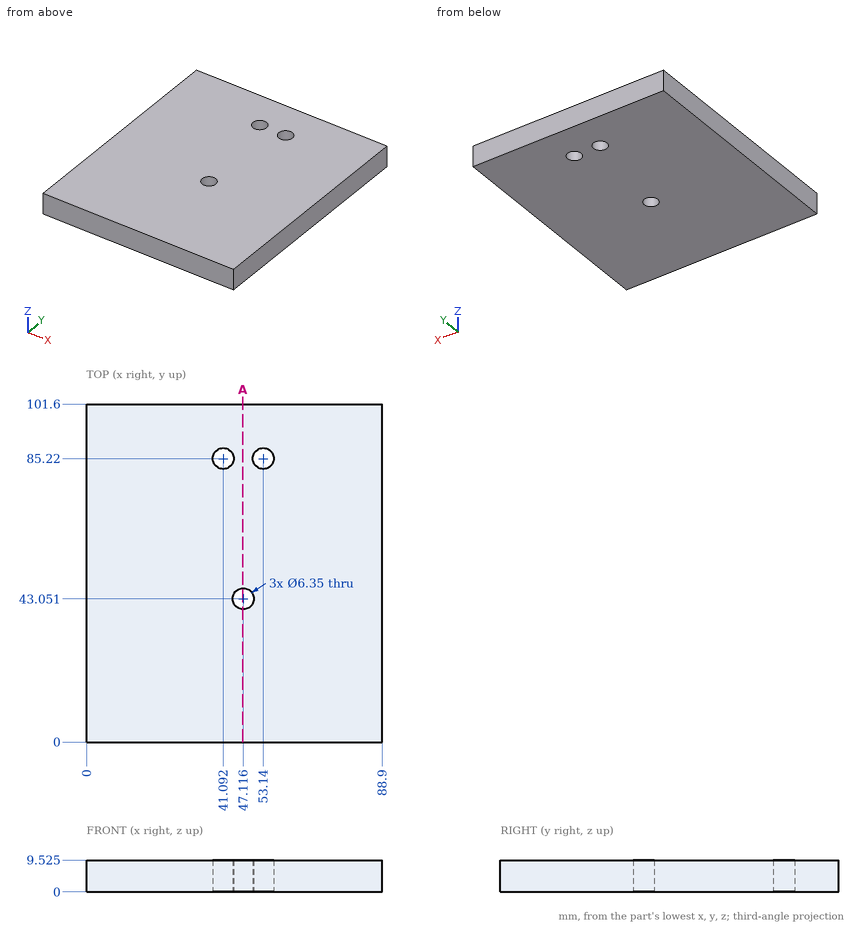
Check sheet for the drawn part. Datum: minimum x, y, z corner. Units: mm. Round coordinates to 2 decimals unless told otherwise and drop trailing zeros. Write each loop counter-clockwise with the first axis right and the second up, starting at its lowest first coordinate (ties: lowest second). Pieces come first, ordered by that corner, then holes. Notation, with made-up numbers: (12.5, 41) -> (58.5, 41) arc R30 ccw to (58.5, 66) -> close; hole circle Ø5 at (-20.75, 74.25). An arc over 180 degrees is marked (long way). Write each question's results on one line, items separated by ' | '. Start each with the question number.
1. Material ranges on probe 1 along X at (y, z) = (85, 4.25) (1 decimal); probe 2 along X at (y, z) = (88, 8.75) (1 decimal); probe 3 along X at (y, z) = (43, 6.5), recorded low to high. Write a range as from..to.
2. Cross-section at A-A (x = 47). Enter the section's corners in (y, z) (1 decimal).
3. Depth check by flat-ended pin: P1, Ø8.5, axis at x = 53.14, y = 85.22, coming from the -Z side. Enter the tip coordinate at first touch or a pass-through.
Solutions:
1) probe 1: x = 0..37.9, 44.3..50, 56.3..88.9 | probe 2: x = 0..39.6, 42.6..51.6, 54.7..88.9 | probe 3: x = 0..43.94, 50.29..88.9
2) outline: (0, 0) -> (39.9, 0) -> (39.9, 9.5) -> (0, 9.5) -> close; (46.2, 0) -> (101.6, 0) -> (101.6, 9.5) -> (46.2, 9.5) -> close
3) P1: stops at z = 0
